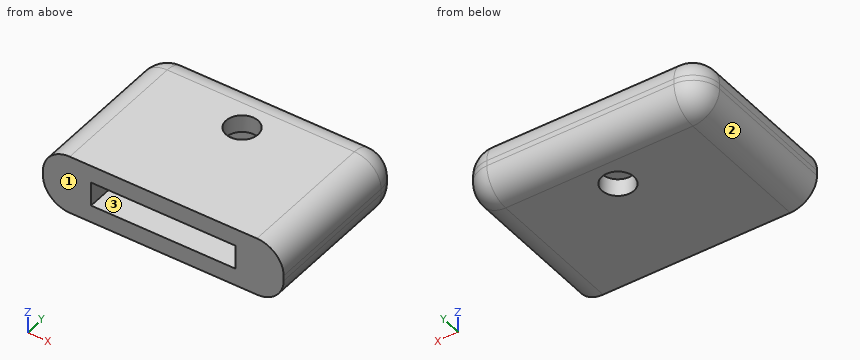
from build123d import *

# Parameters (mm, degrees)
F1_R     = 3
F2_DEPTH = 5.5
F3_DEPTH = 2.25
F4_R     = 5


with BuildPart() as f2:
    # F1 (on Top) → F2 (new body, symmetric)
    with BuildSketch(Plane.XY):
        with BuildLine():
            Line((-22.5, -13), (-13.5, -13))
            Line((-13.5, -13), (-13.5, 8))
            ThreePointArc((-13.5, 8), (-12.0355339059, 11.5355339059), (-8.5, 13))
            Line((-8.5, 13), (8.5, 13))
            ThreePointArc((8.5, 13), (12.0355339059, 11.5355339059), (13.5, 8))
            Line((13.5, 8), (13.5, -13))
            Line((13.5, -13), (22.5, -13))
            Line((22.5, -13), (22.5, 13))
            ThreePointArc((22.5, 13), (21.0355339059, 16.5355339059), (17.5, 18))
            Line((17.5, 18), (-17.5, 18))
            ThreePointArc((-17.5, 18), (-21.0355339059, 16.5355339059), (-22.5, 13))
            Line((-22.5, 13), (-22.5, -13))
        make_face()
        with BuildLine():
            Line((-13.5, 8), (-13.5, -13))
            Line((-13.5, -13), (13.5, -13))
            Line((13.5, -13), (13.5, 8))
            ThreePointArc((13.5, 8), (12.0355339059, 11.5355339059), (8.5, 13))
            Line((8.5, 13), (-8.5, 13))
            ThreePointArc((-8.5, 13), (-12.0355339059, 11.5355339059), (-13.5, 8))
        make_face()
        with Locations((0, 8)):
            Circle(F1_R, mode=Mode.SUBTRACT)
    extrude(amount=F2_DEPTH, both=True)

    # F1 (on Top) → F3 (cut, symmetric)
    with BuildSketch(Plane.XY):
        with BuildLine():
            Line((-13.5, 8), (-13.5, -13))
            Line((-13.5, -13), (13.5, -13))
            Line((13.5, -13), (13.5, 8))
            ThreePointArc((13.5, 8), (12.0355339059, 11.5355339059), (8.5, 13))
            Line((8.5, 13), (-8.5, 13))
            ThreePointArc((-8.5, 13), (-12.0355339059, 11.5355339059), (-13.5, 8))
        make_face()
        with Locations((0, 8)):
            Circle(F1_R, mode=Mode.SUBTRACT)
    extrude(amount=F3_DEPTH, both=True, mode=Mode.SUBTRACT)

    # F4
    f4_edges = [f2.edges().sort_by_distance(p)[0] for p in [
        (-22.5, 0, 5.5),
        (-21.035534, 16.535534, 5.5),
        (0, 18, 5.5),
        (21.035534, 16.535534, 5.5),
        (22.5, 0, 5.5),
        (22.5, 0, -5.5),
    ]]
    fillet(f4_edges, radius=F4_R)


solid = f2.part
Verification items for the finished model (mm, model axes). Face numbers are marked on the shaded views. Give positions to 0.01 mm unless a question says otherwise; leave off trailing zeros. Order: outer loops, then holes, each group sorted by start corner. A loop starts at its lowest first (then second) coordinate and runs counter-clockwise, first axis right, second up. Notation, with made-up numbers: M -23,-26.75 L -9,-26.75 A36 cw -9,12.25 Z; hole C -19,-8.5 d4. An arc over 180 degrees is marked long. Answer as a JSON object with one key per item and string values. Group by question number.
1) Scan lines: line 1 along Z through (x, y) = (-6.5, -4); line 2 along X through (y, z) = (2.5, 0.25); line 3 along X through (y, z) = (7, 4). Record each from-to range of solid material in increasing order. Write a range as [from, to].
2) Mould release check, pull along Z, two halves, no side actions. Record for the marked faces 1, 2 and 3: released by +Z, released by -Z, zero draft, split by the parting line, or undercut.
3) Depth check by flat-ended pin: pin 1 Ø3.5 at (x, z) = (-0.5, -1) entering from -Y; pin 2 Ø5.5 at (x, y) = (0, 8) entering from +Z. Enter the tip coordinate at first touch or a pass-through.
4) Cross-section at D-D (y = 7). Enter the section's corners in (x, z), then the cut area to 3 significant figures.
5) Cross-section at B-B (x = 4.5). Enter the section's corners in (y, z).
6) Cross-section at A-A (x = 0). Enter the section's corners in (y, z).
7) Cross-section at C-C (z = 3). Enter the section's corners in (x, y).
Result sheet:
{
 "1": {"line 1": "z = [-5.5, -2.25], [2.25, 5.5]", "line 2": "x = [-22.5, -13.5], [13.5, 22.5]", "line 3": "x = [-21.07, -2.83], [2.83, 21.07]"},
 "2": {"face 1": "zero draft", "face 2": "released by -Z", "face 3": "undercut"},
 "3": {"pin 1": "stops at y = -13", "pin 2": "passes through"},
 "4": {"outline": "M -22.5,-0.5 A5 ccw -17.5,-5.5 L -2.83,-5.5 L -2.83,-2.25 L -13.5,-2.25 L -13.5,2.25 L -2.83,2.25 L -2.83,5.5 L -17.5,5.5 A5 ccw -22.5,0.5 Z; M 2.83,-5.5 L 17.5,-5.5 A5 ccw 22.5,-0.5 L 22.5,0.5 A5 ccw 17.5,5.5 L 2.83,5.5 L 2.83,2.25 L 13.5,2.25 L 13.5,-2.25 L 2.83,-2.25 Z", "area": "315 mm2"},
 "5": {"outline": "M -13,-5.5 L 13,-5.5 A5 ccw 18,-0.5 L 18,0.5 A5 ccw 13,5.5 L -13,5.5 L -13,2.25 L 13,2.25 L 13,-2.25 L -13,-2.25 Z"},
 "6": {"outline": "M -13,-5.5 L 5,-5.5 L 5,-2.25 L -13,-2.25 Z; M -13,2.25 L 5,2.25 L 5,5.5 L -13,5.5 Z; M 11,-5.5 L 13,-5.5 A5 ccw 18,-0.5 L 18,0.5 A5 ccw 13,5.5 L 11,5.5 L 11,2.25 L 13,2.25 L 13,-2.25 L 11,-2.25 Z"},
 "7": {"outline": "M -21.83,-13 L 21.83,-13 L 21.83,13 A4.33 ccw 17.5,17.33 L -17.5,17.33 A4.33 ccw -21.83,13 Z; hole C 0,8 d6"}
}
